Here's how the part is built. I have some questions about the finished solid (model axes, mm). Face numbers are marked on the shaded views. Give positions to 0.01 mm unless a question says otherwise; leave off trailing zeros. Order: outer loops, then holes, each group sorted by start corner. A loop starts at its lowest first (then second) coordinate and runs counter-clockwise, first axis right, second up. Notation, with made-up numbers: M 56,64 L 67,64 A27 cw 67,80 Z; hole C -5,57.25 d8. An arc over 180 degrees is marked long. One line per item, written item: value. Start each with the question number.
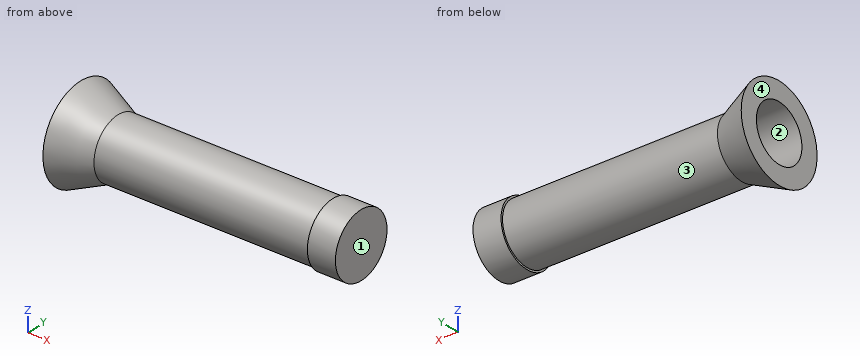
from build123d import *

# Parameters (mm, degrees)
SKETCH2_R          = 15
CUT_EXTRUDE1_DEPTH = 145


with BuildPart() as part:
    # Sketch1 → Revolve1 (revolve)
    with BuildSketch(Plane.XY):
        Polygon((-115, 0), (-135, 9), (-135, -16), (15, -16), (15, 1), (0, 1), (0, 0), align=None)
    revolve(axis=Axis((15, -16, 0), (-1, 0, 0)))

    # Sketch2 → Cut-Extrude1 (cut)
    with BuildSketch(Plane.ZY.offset(135)):
        with Locations((0, -16)):
            Circle(SKETCH2_R)
    extrude(amount=-CUT_EXTRUDE1_DEPTH, mode=Mode.SUBTRACT)


solid = part.part
Item 1: I want a section at A-A on y = -16. Write out the boundary of the cut face in (x, z), plus the area to 3 significant figures.
Item 2: I want a section at B-B on z = 0. Write out the boundary of the cut face in (x, y).
Item 3: Please list where these lines run through material, in increasing order: probe 1 along Y at (x, z) = (-102, 0); probe 2 along Z at (x, y) = (-112, -15.5); probe 3 along Z at (x, y) = (-38, -14). Write a range as [from, to].
Item 4: I want a section at C-C on x = -35.5. Write out the boundary of the cut face in (y, z).
Item 5: Will these pins go through, and if not, where does the flat tip stop? P1, Ø24, axis at y = -14, z = -4, coming from the -X side; P2, Ø12, axis at x = -2.5, z = 11.5, coming from the +Y side; P3, Ø1, axis at x = -113, z = -10.5, coming from the -Y side; P4, Ø1.5, axis at x = -75, z = 11.5, coming from the +Y side.
Item 6: I want a section at D-D on x = -126. Write out the boundary of the cut face in (y, z), plus the area to 3 significant figures.
Item 7: We'd pull the mould along X, two halves only. Please class the marked faces 1, 2, 3 and 4: +X half, -X half, draft (parallel to the pull), parting line (faces both ways), or undercut.
Answer below:
1. outline: M -135,-25 L -115,-16 L 0,-16 L 0,-17 L 15,-17 L 15,17 L 0,17 L 0,16 L -115,16 L -135,25 L -135,15 L 10,15 L 10,-15 L -135,-15 Z
1. area: 660 mm²
2. outline: M -135,-41 L -115,-32 L 0,-32 L 0,-33 L 15,-33 L 15,1 L 0,1 L 0,0 L -115,0 L -135,9 L -135,-1 L 10,-1 L 10,-31 L -135,-31 Z
3. probe 1: y = [-32, -31], [-1, 0]
3. probe 2: z = [-15.99, -14.99], [14.99, 15.99]
3. probe 3: z = [-15.87, -14.87], [14.87, 15.87]
4. outline: C -16,0 d32; hole C -16,0 d30
5. P1: stops at x = -135
5. P2: stops at y = -0.11
5. P3: stops at y = -28.49
5. P4: stops at y = -4.15
6. outline: C -16,0 d41.9; hole C -16,0 d30
6. area: 672 mm²
7. face 1: +X half
7. face 2: draft
7. face 3: undercut
7. face 4: -X half
